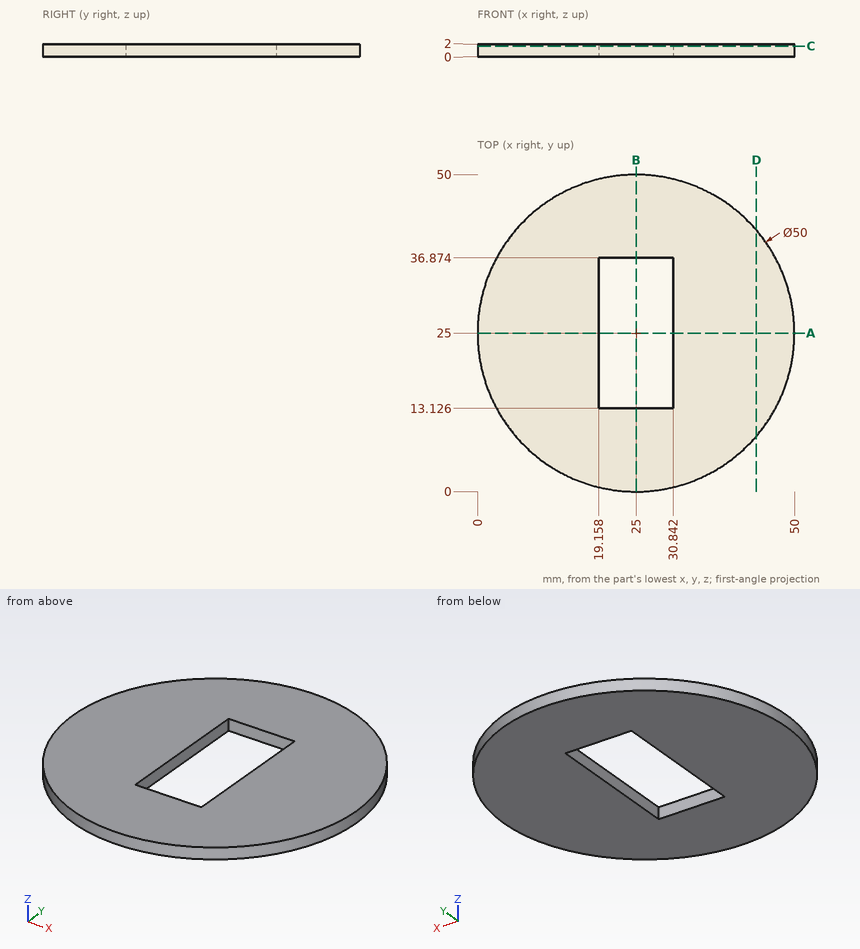
Could you check a few things on this drawing? It's one solid part, dimensions in mm from its lowest x, y, z. Round coordinates to 2 decimals unless told otherwise and drop trailing zeros. Order: outer loops, then holes, each group sorted by start corner. A loop starts at its lowest first (then second) coordinate and runs counter-clockwise, first axis right, second up.
Q1. Imagine slicing it at C-C, the plane z = 1.65. List the corners of the cut face in (x, y) for me (1 decimal), then the cut area to 3 significant figures.
Geometry says:
outline: circle Ø50 at (25, 25); hole (19.2, 13.1) - (30.8, 13.1) - (30.8, 36.9) - (19.2, 36.9) - close
area: 1,690 mm2
Q2. Please list where these lines run through material, in increasing order: probe 1 along X at (y, z) = (14.5, 0.25); probe 2 along X at (y, z) = (19, 0.55); probe 3 along Y at (x, z) = (28.5, 0.9) (1 decimal).
Geometry says:
probe 1: x = 2.31 to 19.16, 30.84 to 47.69
probe 2: x = 0.73 to 19.16, 30.84 to 49.27
probe 3: y = 0.2 to 13.1, 36.9 to 49.8
Q3. Imagine slicing it at A-A, the plane y = 25. List the corners of the cut face in (x, z) for me.
Geometry says:
outline: (0, 0) - (19.16, 0) - (19.16, 2) - (0, 2) - close; (30.84, 0) - (50, 0) - (50, 2) - (30.84, 2) - close
Q4. Imagine slicing it at B-B, the plane x = 25. List the corners of the cut face in (y, z) for me (1 decimal).
Geometry says:
outline: (0, 0) - (13.1, 0) - (13.1, 2) - (0, 2) - close; (36.9, 0) - (50, 0) - (50, 2) - (36.9, 2) - close
Q5. Imagine slicing it at D-D, the plane x = 44. List the corners of the cut face in (y, z) for me.
Geometry says:
outline: (8.75, 0) - (41.25, 0) - (41.25, 2) - (8.75, 2) - close
Q6. I'm going to push flat-ended pins straight in: P1, Ø4, axis at x = 20, y = 29, coming from the -Z side; P2, Ø0.6, axis at x = 22.5, z = 1, coming from the +Y side; P3, Ø0.6, axis at y = 20, z = 1.5, coming from the -X side (1 decimal). Where does each tip first touch, or does it pass through?
Geometry says:
P1: stops at z = 0
P2: stops at y = 49.9
P3: stops at x = 0.4
